from build123d import *

# Parameters (mm, degrees)
F0_W      = 254
F0_H      = 254
F1_DEPTH  = 254
F6_DEPTH  = 254
F8_DEPTH  = 254
F4_DEPTH  = 254.000008
F10_DEPTH = 254


with BuildPart() as f1:
    # F0 (on Front) → F1 (new body)
    with BuildSketch(Plane.XZ):
        with Locations((127, 127)):
            Rectangle(F0_W, F0_H)
    extrude(amount=F1_DEPTH)

    # F2 (on Front) → F6 (cut, through all)
    with BuildSketch(Plane.XZ):
        Polygon((0, 0), (127, 254), (0, 254), align=None)
    extrude(amount=F6_DEPTH, mode=Mode.SUBTRACT)

    # F7 (on Front) → F8 (cut, through all)
    with BuildSketch(Plane.XZ):
        Polygon((254, 254), (127, 254), (254, 0), align=None)
    extrude(amount=F8_DEPTH, mode=Mode.SUBTRACT)

    # F9 (on Right) → F4 (cut)
    with BuildSketch(Plane.YZ):
        Polygon((-254, 254), (-254, 0), (-127, 254), align=None)
    extrude(amount=F4_DEPTH, mode=Mode.SUBTRACT)

    # F5 (on Right) → F10 (cut)
    with BuildSketch(Plane.YZ):
        Polygon((0, 254), (-127, 254), (0, 0), align=None)
    extrude(amount=F10_DEPTH, mode=Mode.SUBTRACT)


solid = f1.part
The listing builds one solid part. Answer for the finished solid, in the listing's coordinates (mm). Coordinates: 2 decimals unless noted, no trailing zeros. Order: outer loops, then holes, each group sorted by start corner. A loop starts at its lowest first (then second) coordinate and runs counter-clockwise, first axis right, second up. Notation, with made-up numbers: (46.25, 25) -> (50.25, 25) arc R23 cw to (50.25, 42) -> close; hole circle Ø11 at (8, 58.5). An arc over 180 degrees is marked (long way). Answer in a Markdown table with one row per item. Add a question column.
Item 1: Find section A-A (y = -161.5). Write down the section's boundary in (x, z), then the cut area to 3 significant figures.
Item 2: Find the intervals of material crossed by L1, parallel to Z at x = 66.5, y = -39; L2, parallel to Y at x = 55.5, z = 89; L3, parallel to X at y = -196.5, z = 44, in increasing order. Write a range as from..to.
Item 3: Find section B-B (x = 82). Write down the section's boundary in (y, z), then the cut area to 3 significant figures.
Item 4: Each of these flat-tipped pins is pushed along its axis until it touches: P1, Ø3, axis at y = -58.5, z = 69.5, coming from the +X side; P2, Ø10, axis at x = 92.5, z = 76, coming from the -Y side; P3, Ø10, axis at x = 205.5, z = 101, coming from the -Y side. Where does it stop, or does it pass through?
Result set:
| question | item | result |
|---|---|---|
| 1 | outline | (0, 0) -> (254, 0) -> (161.5, 185) -> (92.5, 185) -> close |
| 1 | area | 29,900 mm² |
| 2 | L1 | z = 0..78 |
| 2 | L2 | y = -209.5..-44.5 |
| 2 | L3 | x = 22..232 |
| 3 | outline | (-254, 0) -> (0, 0) -> (-82, 164) -> (-172, 164) -> close |
| 3 | area | 28,200 mm² |
| 4 | P1 | stops at x = 220 |
| 4 | P2 | stops at y = -218.5 |
| 4 | P3 | stops at y = -206 |
